from build123d import *

# Parameters (mm, degrees)
BOSS_EXTRUDE1_DEPTH = 5
SKETCH3_W           = 8
SKETCH3_H           = 4
BOSS_EXTRUDE2_DEPTH = 3
FILLET1_START       = -3.841593316
FILLET1_DEPTH       = 8
CUT_EXTRUDE1_START  = -10
CUT_EXTRUDE1_DEPTH  = 10
FILLET2_R           = 3
SKETCH6_R           = 1.25
CUT_EXTRUDE2_DEPTH  = 5
CUT_EXTRUDE3_START  = -5
SKETCH7_R           = 1.25
CUT_EXTRUDE3_DEPTH  = 5


with BuildPart() as part:
    # Sketch1 → Boss-Extrude1 (new body)
    with BuildSketch(Plane(origin=(0, 0, 0), x_dir=(1, 0, 0), z_dir=(0, 1, 0))):
        with BuildLine():
            Line((-30, 0), (30, 0))
            ThreePointArc((30, 0), (0, 30), (-30, 0))
        make_face()
    extrude(amount=BOSS_EXTRUDE1_DEPTH)

    # Sketch3 → Boss-Extrude2 (add)
    with BuildSketch(Plane(origin=(0, 5, 0), x_dir=(1, 0, 0), z_dir=(0, 1, 0))):
        with Locations((0.158406684, 24.731666579)):
            Rectangle(SKETCH3_W, SKETCH3_H)
    extrude(amount=BOSS_EXTRUDE2_DEPTH)

    # Fillet1: read off the stored shape, not the designer's step
    # Fillet1 outline → Fillet1 (cut)
    with BuildSketch(Plane.YZ.offset(FILLET1_START)):
        with BuildLine():
            Line((8, -22.731666579), (5, -22.731666579))
            add(Edge.make_bspline(
                [(5, -22.731666579), (8, -23.506263249), (8, -26.604649926)],
                knots=[0, 0, 0, 1, 1, 1], degree=2, weights=[1, 0.057495957, 1]))
            Line((8, -26.604649926), (8, -22.731666579))
        make_face()
    extrude(amount=FILLET1_DEPTH, mode=Mode.SUBTRACT)

    # Sketch5 → Cut-Extrude1 (cut)
    with BuildSketch(Plane(origin=(0, 5, 0), x_dir=(1, 0, 0), z_dir=(0, 1, 0)).offset(CUT_EXTRUDE1_START)):
        with BuildLine():
            Line((-21.580398915, 0), (-21.580398915, 5))
            Line((-21.580398915, 5), (-29.580398915, 5))
            ThreePointArc((-29.580398915, 5), (-29.894915684, 2.508787808), (-30, 0))
            Line((-30, 0), (-21.580398915, 0))
        make_face()
        with BuildLine():
            Line((21.580398915, 5), (29.580398915, 5))
            ThreePointArc((29.580398915, 5), (29.894915684, 2.508787808), (30, 0))
            Line((30, 0), (21.580398915, 0))
            Line((21.580398915, 0), (21.580398915, 5))
        make_face()
    extrude(amount=CUT_EXTRUDE1_DEPTH, mode=Mode.SUBTRACT)

    # Fillet2
    fillet2_edges = [part.edges().sort_by_distance(p)[0] for p in [
        (0, 5, 0),
    ]]
    fillet(fillet2_edges, radius=FILLET2_R)

    # Sketch6 → Cut-Extrude2 (cut)
    with BuildSketch(Plane(origin=(21.580398915, 0, 0), x_dir=(0, 0, -1), z_dir=(1, 0, 0))):
        with Locations((3, 2.25)):
            Circle(SKETCH6_R)
    extrude(amount=-CUT_EXTRUDE2_DEPTH, mode=Mode.SUBTRACT)

    # Sketch7 → Cut-Extrude3 (cut)
    with BuildSketch(Plane.ZY.offset(21.580398915).offset(CUT_EXTRUDE3_START)):
        with Locations(Location((-3, 2.25, 0), (0, 0, 180))):
            Circle(SKETCH7_R)
    extrude(amount=CUT_EXTRUDE3_DEPTH, mode=Mode.SUBTRACT)


solid = part.part
Build history of the part. All positions in model axes, mm. A direction names the side the tool comes from. Round coordinates to 2 decimals unless told otherwise and drop trailing zeros. Write each loop counter-clockwise with the first axis right and the second up, starting at its lowest first coordinate (ties: lowest second). Pieces come first, ordered by that corner, then holes. Notation, with made-up numbers: (66.5, 23.25) - (113.5, 23.25) arc R35 ccw to (113.5, 60.25) - close; hole circle Ø6 at (-26, -18.5). An arc over 180 degrees is marked (long way). One line per question, with ' | ' between items.
1. Drop flat-ended pins along their axis: pin 1 Ø1.5 at (y, z) = (3.5, -5.5) entering from +X; pin 2 Ø1 at (x, z) = (2, -10.5) entering from +Y; pin 3 Ø2.5 at (x, y) = (-26.5, 2) entering from +Z; pin 4 Ø1.5 at (x, y) = (1.5, 7) entering from -Z. Give the stop position or say it passes through.
Results are:
pin 1: x = 29.58 | pin 2: y = 5 | pin 3: z = -5 | pin 4: z = -26.73
2. Drill centre lines: line 1 along Y through (x, z) = (3, -9); line 2 along Z through (x, y) = (-25, 4.5); line 3 along Z through (x, y) = (-18.3, 2.25). Where is each one in solid material? Low to high. Write a range as from..to.
Results are:
line 1: 0..5 | line 2: -16.58..-5 | line 3: -23.77..-4.25, -1.75..-0.01
3. Mould opens along Z. For faces 6 (the face through (-16.58, 2, -3)), 7 (the face through (16.58, 2, -3)), 8 (the face through (0, 5, -14)), 9 (the face through (-26, 2, -5)) say: released by +Z, released by -Z, zero draft, split by the parting line, or undercut.
Results are:
face 6: undercut | face 7: undercut | face 8: zero draft | face 9: released by +Z
4. Tool access for faces 1 (the face through (-3.842, 6, -25)), 2 (the face through (19, 3, -4)), 3 (the face through (26, 2, -5)), 4 (the face through (-19, 1.9, -4.2)), 5 (the face through (0, 6, -26.732)): list every direction of +Z, -Z, +X, -X, +Y, -Y with a clear straight run to the whole face (end or side of a thin tool).
Results are:
face 1: +Z, -Z, -X, +Y | face 2: +X | face 3: +Z, +X, +Y, -Y | face 4: -X | face 5: -Z, +X, -X, +Y
5. Band-saw the part on B-B, the plane z = -15.5. Write the cut outline in (x, y), and give its area (3 significant figures).
Results are:
outline: (-25.69, 0) - (25.69, 0) - (25.69, 5) - (-25.69, 5) - close | area: 257 mm^2
6. Band-saw the part on A-A, the plane x = 11. Write the cut outline in (y, z), and give its area (3 significant figures).
Results are:
outline: (0, -27.91) - (5, -27.91) - (5, -3) arc R3 ccw to (2, 0) - (0, 0) - close | area: 138 mm^2
